Geometry: final body of the model. Coordinates: model frame, mm. A direction names the side the tool comes from. Give positions to 0.01 mm unless a question says otherwise; leave off trailing zeros. Loops run counter-clockwise (first coordinate to the right, second up) from the corner with the lowest first, then second, coordinate; pieces in that order, holes last. Notation, with made-up numbers: M -37,87 L -14,87 A22 cw -14,110 Z; hole C 22,33.25 d4. An arc over 180 degrees is marked long. Put each result on its own line as item: value.
```python
from build123d import *

# Parameters (mm, degrees)
SKETCH_1_R             = 28.5
EXTRUDE_1_DEPTH        = 45
SKETCH_2_R             = 17.5
EXTRUDE_2_DEPTH        = 1
SKETCH_3_R             = 1
SKETCH_3_R_2           = 1.5
CUT_EXTRUDE_1_DEPTH    = 5
HOLE_WIZARD_M3_1_D     = 2.5
HOLE_WIZARD_M3_1_DEPTH = 5
HOLE_WIZARD_M3_1_TIP   = 0.751075774
SKETCH_7_R             = 1
SKETCH_7_R_2           = 2
CUT_EXTRUDE_2_DEPTH    = 5
HOLE_WIZARD_M3_2_D     = 2.5
HOLE_WIZARD_M3_2_DEPTH = 7
HOLE_WIZARD_M3_2_TIP   = 0.751075774
SKETCH_10_R            = 1
CUT_EXTRUDE_3_DEPTH    = 4
HOLE_WIZARD_M3_3_D     = 2.5
HOLE_WIZARD_M3_3_DEPTH = 4
HOLE_WIZARD_M3_3_TIP   = 0.751075774
SKETCH_12_W            = 4.5
SKETCH_12_H            = 13.5
EXTRUDE_3_DEPTH        = 16.4
SKETCH_14_R            = 2.127458751
SKETCH_14_R_2          = 0.821166135
EXTRUDE_4_DEPTH        = 6


with BuildPart() as part:
    # 草图1 → 凸台-拉伸1 (new body)
    with BuildSketch(Plane.XY):
        Circle(SKETCH_1_R)
    extrude(amount=EXTRUDE_1_DEPTH)

    # 草图2 → 凸台-拉伸2 (add)
    with BuildSketch(Plane.XY.offset(45)):
        Circle(SKETCH_2_R)
    extrude(amount=EXTRUDE_2_DEPTH)

    # 草图3 → 切除-拉伸1 (cut)
    with BuildSketch(Plane.XY.offset(45)):
        with Locations((0, 25)):
            Circle(SKETCH_3_R)
        with Locations((21.650635095, 12.5)):
            Circle(SKETCH_3_R)
        with Locations((21.650635095, -12.5)):
            Circle(SKETCH_3_R)
        with Locations((0, -25)):
            Circle(SKETCH_3_R)
        with Locations((-21.650635095, -12.5)):
            Circle(SKETCH_3_R)
        with Locations((-21.650635095, 12.5)):
            Circle(SKETCH_3_R)
        with Locations((-6.470476128, -24.148145657)):
            Circle(SKETCH_3_R_2)
        with Locations((6.470476128, 24.148145657)):
            Circle(SKETCH_3_R_2)
    extrude(amount=-CUT_EXTRUDE_1_DEPTH, mode=Mode.SUBTRACT)

    # M3 螺纹孔1
    with Locations(Plane.XY.offset(45)):
        with Locations((-21.650635095, 12.5), (0, 25), (21.650635095, 12.5), (21.650635095, -12.5), (0, -25), (-21.650635095, -12.5)):
            Hole(HOLE_WIZARD_M3_1_D / 2, depth=HOLE_WIZARD_M3_1_DEPTH)
            with Locations((0, 0, -(HOLE_WIZARD_M3_1_DEPTH + HOLE_WIZARD_M3_1_TIP / 2))):  # 118° drill point
                Cone(0, HOLE_WIZARD_M3_1_D / 2, HOLE_WIZARD_M3_1_TIP, mode=Mode.SUBTRACT)

    # 草图7 → 切除-拉伸2 (cut)
    with BuildSketch(Plane.XY.offset(46)):
        with Locations((0, 13.5)):
            Circle(SKETCH_7_R)
        with Locations((11.691342951, 6.75)):
            Circle(SKETCH_7_R)
        with Locations((11.691342951, -6.75)):
            Circle(SKETCH_7_R)
        with Locations((0, -13.5)):
            Circle(SKETCH_7_R)
        with Locations((-11.691342951, -6.75)):
            Circle(SKETCH_7_R)
        with Locations((-11.691342951, 6.75)):
            Circle(SKETCH_7_R)
        with Locations((12.15, 0)):
            Circle(SKETCH_7_R_2)
        with Locations((-6.075, -10.522208656)):
            Circle(SKETCH_7_R_2)
        with Locations((-6.075, 10.522208656)):
            Circle(SKETCH_7_R_2)
    extrude(amount=-CUT_EXTRUDE_2_DEPTH, mode=Mode.SUBTRACT)

    # M3 螺纹孔2
    with Locations(Plane.XY.offset(46)):
        with Locations((-11.691342951, 6.75), (0, 13.5), (11.691342951, 6.75), (11.691342951, -6.75), (0, -13.5), (-11.691342951, -6.75)):
            Hole(HOLE_WIZARD_M3_2_D / 2, depth=HOLE_WIZARD_M3_2_DEPTH)
            with Locations((0, 0, -(HOLE_WIZARD_M3_2_DEPTH + HOLE_WIZARD_M3_2_TIP / 2))):  # 118° drill point
                Cone(0, HOLE_WIZARD_M3_2_D / 2, HOLE_WIZARD_M3_2_TIP, mode=Mode.SUBTRACT)

    # 草图10 → 切除-拉伸3 (cut)
    with BuildSketch(Plane(origin=(0, 0, 0), x_dir=(-1, 0, 0), z_dir=(0, 0, -1))):
        with Locations((-4.5, 18.459414942)):
            Circle(SKETCH_10_R)
        with Locations((18.459414942, 4.5)):
            Circle(SKETCH_10_R)
        with Locations((4.5, -18.459414942)):
            Circle(SKETCH_10_R)
        with Locations((-18.459414942, -4.5)):
            Circle(SKETCH_10_R)
    extrude(amount=-CUT_EXTRUDE_3_DEPTH, mode=Mode.SUBTRACT)

    # M3 螺纹孔3
    with Locations(Plane(origin=(4.5, 18.459414942, 0), x_dir=(-1, 0, 0), z_dir=(0, 0, -1))):
        with Locations((0, 0), (-13.959414942, -22.959414942), (9, -36.918829884), (22.959414942, -13.959414942)):
            Hole(HOLE_WIZARD_M3_3_D / 2, depth=HOLE_WIZARD_M3_3_DEPTH)
            with Locations((0, 0, -(HOLE_WIZARD_M3_3_DEPTH + HOLE_WIZARD_M3_3_TIP / 2))):  # 118° drill point
                Cone(0, HOLE_WIZARD_M3_3_D / 2, HOLE_WIZARD_M3_3_TIP, mode=Mode.SUBTRACT)

    # 草图12 → 凸台-拉伸3 (add)
    with BuildSketch(Plane(origin=(10.411631287, 6.330312934, 0), x_dir=(0, 0, -1), z_dir=(0.854460947, 0.51951563, 0))):
        with Locations((-3.75, 0)):
            Rectangle(SKETCH_12_W, SKETCH_12_H)
    extrude(amount=EXTRUDE_3_DEPTH)

    # 草图14 → 凸台-拉伸4 (add)
    with BuildSketch(Plane(origin=(24.424790822, 14.850369263, 0), x_dir=(0, 0, -1), z_dir=(0.854460947, 0.51951563, 0))):
        with Locations((-3.791208739, 4.492201758)):
            Circle(SKETCH_14_R)
        with Locations((-3.791208739, -0.213214329)):
            Circle(SKETCH_14_R)
        with Locations((-4.780701919, -5.253978847)):
            Circle(SKETCH_14_R_2)
        with Locations((-2.591443579, -5.253978847)):
            Circle(SKETCH_14_R_2)
    extrude(amount=EXTRUDE_4_DEPTH)


solid = part.part
```
Item 1: Section B-B on z = 34. Output: boundary loops of the cut face in (x, y), then the cut area to 3 significant figures.
Output values:
outline: C 0,0 d57
area: 2,550 mm²
Item 2: Section A-A on x = 7. Output: boundary loops of the cut face in (y, z), then the cut area to 3 significant figures.
Output values:
outline: M -27.63,0 L 27.63,0 L 27.63,45 L 25.55,45 L 25.55,40 L 22.74,40 L 22.74,45 L 16.04,45 L 16.04,46 L -16.04,46 L -16.04,45 L -27.63,45 Z
area: 2,500 mm²
Item 3: Set-up query: faces 4 (the cylindrical face through (-5.421, -17.615, 2.028)), 5 (the cylindrical face through (29.66, 11.93, 3.41)), 6 (the flat face through (-6, -24, 40)). Return all of +Z, -Z, +X, -X, +Y, -Y with unobstructed straight access to the full face (end or side cutting, diameter ignored); none if empty.
Output values:
face 4: -Z
face 5: none
face 6: +Z
Item 4: Section D-D on x = 15.5. Output: boundary loops of the cut face in (y, z).
Output values:
outline: M -23.92,0 L 23.92,0 L 23.92,45 L 8.12,45 L 8.12,46 L -8.12,46 L -8.12,45 L -23.92,45 Z
Item 5: Section C-C on y = -20.5. Output: boundary loops of the cut face in (x, z), then the cut area to 3 significant figures.
Output values:
outline: M -19.8,0 L 19.8,0 L 19.8,45 L -19.8,45 Z
area: 1,780 mm²
Item 6: Line query: probe 1 along Y at (x, z) = (0, 41.6); probe 2 along X at (y, z) = (12, 42) (3 decimals); probe 3 along X at (y, z) = (6.75, 42.75). Output: solid intervals per line, ascending. Write a range as [from, to].
Output values:
probe 1: [-28.5, -26.25], [-23.75, -14.75], [-12.25, 12.25], [14.75, 23.75], [26.25, 28.5]
probe 2: [-25.851, -22.796], [-20.505, -7.423], [-4.727, 20.505], [22.796, 25.851]
probe 3: [-27.69, -12.94], [-10.44, 10.44], [12.94, 27.69]
Item 7: Mould query, pull axis X, two halves, no side actions, for faces 1 (the conical face through (-18.24, 4.51, 4.62)), 2 (the flat face through (12, 13, 45)), 3 (the flat face through (27.202, 21.831, 3.821)). Classes: pulls with the +X half, pulls with the -X half, needs draft (parallel to the pull), parting line crosses it, or undercut.
Output values:
face 1: undercut
face 2: needs draft
face 3: pulls with the +X half
Item 8: Pin query (flat end, axial travel): pin 1 Ø10 at (x, z) = (-8, 18) entering from -Y; pin 2 Ø2 at (x, z) = (2, 29) entering from -Y; pin 3 Ø2.5 at (x, y) = (-6, -23.5) entering from +Z. Return the tip coordinate at first contact, or that it passes through.
Output values:
pin 1: y = -28.34
pin 2: y = -28.48
pin 3: z = 45
